Read the model definition and answer for the solid it produces. Units are mm, in the model's axes. Face numbers are marked on the shaded views. Round coordinates to 2 decimals unless told otherwise and drop trailing zeros. Write each loop counter-clockwise with the first axis right and the second up, starting at its lowest first coordinate (ties: lowest second). Pieces come first, ordered by that corner, then holes. Notation, with made-up numbers: (79.5, 45.25) -> (127.5, 45.25) arc R20 ccw to (127.5, 59.25) -> close; hole circle Ø5 at (47, 26.25). An arc over 180 degrees is marked (long way). Return JSON: item names as keys, results as strings. Group by question number.
(1) A cutting plane is placed at D-D on x = -3.5. Give the vertices of the cut face in (y, z), then the cut area to 3 significant figures.
(2) A cutting plane is placed at C-C on z = 10.5. Give the vertices of the cut face in (x, y).
(3) Straight lines are drawn through the part: line 1 (Z direction, x = -3.75, y = 2.75); line 2 (X direction, y = 0, z = 19.75); line 3 (Z direction, x = 1.5, y = 1). For each, find the intervals that lie inside material, in ascending order.
(4) A cutting plane is placed at B-B on y = -0.25. Give the vertices of the cut face in (x, z).
(5) A cutting plane is placed at A-A on x = 0.25. Give the vertices of the cut face in (y, z), then the cut area to 3 significant figures.
(6) Given pin 1 (3 mm diameter, centred on x = -1, y = 0, fed in from +Z); pin 2 (2 mm diameter, centred on x = 0, z = 17.5, fed in from -Y); pin 3 (6 mm diameter, centred on y = 4, z = 11.5, fed in from -X); pin 4 (0.8 mm diameter, centred on y = -1, z = 20.5, fed in from -X), each flat-ended and moving along its own axis, determine where each tip first touches the part or whether it passes through.
(7) The mould has two halves that part along Y. Classify the marked faces 1 and 2: released by +Y, released by -Y, zero draft, split by the parting line, or undercut.
```python
from build123d import *

# Parameters (mm, degrees)
F1_DEPTH = 21
F2_DEPTH = 20
F3_DEPTH = 2
F4_DEPTH = 20.25


with BuildPart() as f1:
    # F0 (on Top) → F1 (new body)
    with BuildSketch(Plane.XY):
        with BuildLine():
            ThreePointArc((0, 4.25), (-3.005204, 3.005204), (-4.25, 0))
            ThreePointArc((-4.25, 0), (-3.005204, -3.005204), (0, -4.25))
            ThreePointArc((0, -4.25), (3.005204, -3.005204), (4.25, 0))
            ThreePointArc((4.25, 0), (3.005204, 3.005204), (0, 4.25))
        make_face()
        Polygon((1.25, -3.85), (-1.25, -3.85), (-1.25, 0.15), (-2.75, 0.15), (0, 3.85), (2.75, 0.15), (1.25, 0.15), align=None, mode=Mode.SUBTRACT)
    extrude(amount=F1_DEPTH)

    # F0 (on Top) → F2 (join)
    with BuildSketch(Plane.XY):
        with BuildLine():
            ThreePointArc((4.75, 0), (3.358757, 3.358757), (0, 4.75))
            ThreePointArc((0, 4.75), (-3.358757, 3.358757), (-4.75, 0))
            ThreePointArc((-4.75, 0), (-3.358757, -3.358757), (0, -4.75))
            ThreePointArc((0, -4.75), (3.358757, -3.358757), (4.75, 0))
        make_face()
        with BuildLine():
            ThreePointArc((0, -4.25), (-3.005204, -3.005204), (-4.25, 0))
            ThreePointArc((-4.25, 0), (-3.005204, 3.005204), (0, 4.25))
            ThreePointArc((0, 4.25), (3.005204, 3.005204), (4.25, 0))
            ThreePointArc((4.25, 0), (3.005204, -3.005204), (0, -4.25))
        make_face(mode=Mode.SUBTRACT)
    extrude(amount=F2_DEPTH)

    # F0 (on Top) → F3 (join)
    with BuildSketch(Plane.XY):
        with BuildLine():
            ThreePointArc((-5.75, 0), (-4.065864, -4.065864), (0, -5.75))
            ThreePointArc((0, -5.75), (4.065864, -4.065864), (5.75, 0))
            ThreePointArc((5.75, 0), (4.065864, 4.065864), (0, 5.75))
            ThreePointArc((0, 5.75), (-4.065864, 4.065864), (-5.75, 0))
        make_face()
        with BuildLine():
            ThreePointArc((-4.75, 0), (-3.358757, 3.358757), (0, 4.75))
            ThreePointArc((0, 4.75), (3.358757, 3.358757), (4.75, 0))
            ThreePointArc((4.75, 0), (3.358757, -3.358757), (0, -4.75))
            ThreePointArc((0, -4.75), (-3.358757, -3.358757), (-4.75, 0))
        make_face(mode=Mode.SUBTRACT)
    extrude(amount=F3_DEPTH)

    # F0 (on Top) → F4 (join)
    with BuildSketch(Plane.XY):
        Polygon((-1.25, 0.15), (-1.25, -3.85), (1.25, -3.85), (1.25, 0.15), (2.75, 0.15), (0, 3.85), (-2.75, 0.15), align=None)
    extrude(amount=F4_DEPTH)


solid = f1.part
```
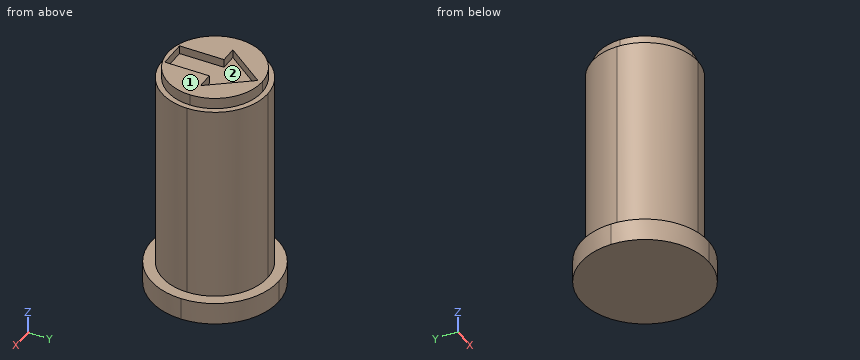
Checks:
{
 "1": {"outline": "(-4.56, 0) -> (4.56, 0) -> (4.56, 2) -> (3.21, 2) -> (3.21, 20) -> (2.41, 20) -> (2.41, 21) -> (-2.41, 21) -> (-2.41, 20) -> (-3.21, 20) -> (-3.21, 2) -> (-4.56, 2) -> close", "area": "139 mm^2"},
 "2": {"outline": "(-4.75, 0) arc R4.75 ccw to (0, -4.75) arc R4.75 ccw to (4.75, 0) arc R4.75 ccw to (0, 4.75) arc R4.75 ccw to start"},
 "3": {"line 1": "z = 0 to 20", "line 2": "x = -4.75 to 4.75", "line 3": "z = 0 to 20.25"},
 "4": {"outline": "(-5.74, 0) -> (5.74, 0) -> (5.74, 2) -> (4.74, 2) -> (4.74, 20) -> (4.24, 20) -> (4.24, 21) -> (1.25, 21) -> (1.25, 20.25) -> (-1.25, 20.25) -> (-1.25, 21) -> (-4.24, 21) -> (-4.24, 20) -> (-4.74, 20) -> (-4.74, 2) -> (-5.74, 2) -> close"},
 "5": {"outline": "(-5.74, 0) -> (5.74, 0) -> (5.74, 2) -> (4.74, 2) -> (4.74, 20) -> (4.24, 20) -> (4.24, 21) -> (3.51, 21) -> (3.51, 20.25) -> (-3.85, 20.25) -> (-3.85, 21) -> (-4.24, 21) -> (-4.24, 20) -> (-4.74, 20) -> (-4.74, 2) -> (-5.74, 2) -> close", "area": "197 mm^2"},
 "6": {"pin 1": "stops at z = 21", "pin 2": "stops at y = -4.75", "pin 3": "stops at x = -4.64", "pin 4": "stops at x = -4.21"},
 "7": {"face 1": "zero draft", "face 2": "undercut"}
}
